Geometry check sheet. Reference: the model listing, model coordinates, mm. A direction names the side the tool comes from. Round coordinates to 2 decimals unless told otherwise and drop trailing zeros. Write each loop counter-clockwise with the first axis right and the second up, starting at its lowest first coordinate (ties: lowest second). Pieces come first, ordered by that corner, then holes.
from build123d import *

# Parameters (mm, degrees)
PAD008_DEPTH    = 3.6
SKETCH034_W     = 6
SKETCH034_H     = 14
SKETCH034_H_2   = 10
POCKET014_DEPTH = 5
FILLET007_R     = 2
SKETCH035_R     = 2.1
POCKET019_DEPTH = 5
SKETCH032_R     = 1.325
POCKET020_DEPTH = 5
SKETCH033_R     = 1.6
HOLE004_DEPTH   = 25
FILLET010_R     = 0.5
POCKET043_DEPTH = 1


with BuildPart() as part:
    # Sketch031 → Pad008 (new body)
    with BuildSketch(Plane.XY):
        Polygon((-12.75, 0), (-12.75, -5), (-12.75, -54), (12.75, -54), (12.75, -5), (12.75, 0), align=None)
    extrude(amount=PAD008_DEPTH)

    # Sketch034 (on Face4 of Pad008) → Pocket014 (cut)
    with BuildSketch(Plane.XY.offset(3.6)):
        with Locations((0, -47)):
            Rectangle(SKETCH034_W, SKETCH034_H)
        with Locations((0, -5)):
            Rectangle(SKETCH034_W, SKETCH034_H_2)
    extrude(amount=-POCKET014_DEPTH, mode=Mode.SUBTRACT)

    # Fillet007
    fillet007_edges = [part.edges().sort_by_distance(p)[0] for p in [
        (-3, -10, 1.8),
        (3, -10, 1.8),
        (3, -40, 1.8),
        (-3, -40, 1.8),
    ]]
    fillet(fillet007_edges, radius=FILLET007_R)

    # Sketch035 (on Face4 of Pad008) → Pocket019 (cut)
    with BuildSketch(Plane.XY.offset(3.6)):
        with Locations((0, -30)):
            Circle(SKETCH035_R)
    extrude(amount=-POCKET019_DEPTH, mode=Mode.SUBTRACT)

    # Sketch032 (on Face4 of Pad008) → Pocket020 (cut)
    with BuildSketch(Plane.XY.offset(3.6)):
        with Locations((-5.7, -24.35)):
            Circle(SKETCH032_R)
        with Locations((5.7, -24.35)):
            Circle(SKETCH032_R)
        with Locations((5.7, -35.65)):
            Circle(SKETCH032_R)
        with Locations((-5.7, -35.65)):
            Circle(SKETCH032_R)
    extrude(amount=-POCKET020_DEPTH, mode=Mode.SUBTRACT)

    # Sketch033 (on Face4 of Pad008) → Hole004 (cut)
    with BuildSketch(Plane.XY.offset(3.6)):
        with Locations((-8, -15)):
            Circle(SKETCH033_R)
        with Locations((8, -15)):
            Circle(SKETCH033_R)
        with Locations((-8, -45)):
            Circle(SKETCH033_R)
        with Locations((8, -45)):
            Circle(SKETCH033_R)
    extrude(amount=-HOLE004_DEPTH, mode=Mode.SUBTRACT)

    # Fillet010
    fillet010_edges = [part.edges().sort_by_distance(p)[0] for p in [
        (-12.75, 0, 1.8),
        (-12.75, -54, 1.8),
        (12.75, 0, 1.8),
        (12.75, -54, 1.8),
    ]]
    fillet(fillet010_edges, radius=FILLET010_R)

    # Sketch098 (on Face31 of Fillet010) → Pocket043 (cut)
    with BuildSketch(Plane.XY.offset(3.6)):
        with BuildLine():
            ThreePointArc((5.7, -21.35), (2.7, -24.35), (5.7, -27.35))
            Line((5.7, -27.35), (12.75, -27.35))
            Line((12.75, -21.35), (12.75, -27.35))
            Line((5.7, -21.35), (12.75, -21.35))
        make_face()
    extrude(amount=-POCKET043_DEPTH, mode=Mode.SUBTRACT)


solid = part.part
1. Access from +Z, -Z, +X, -X, +Y, -Y to the whole of each face (thin tool, end or side, straight path). Record for faces 4 (the face through (0, -40, 2)), 5 (the face through (0, -10, 2)), 6 (the face through (8, 0, 2)).
2. Section check B-B (y = -30). Record the cut outline in (x, z).
3. Section check C-C (x = 0). Record the cut outline in (y, z).
4. Section check D-D (z = 0.95). State how many separate pieces and enclosed holes the cut face has, plus the area to 3 significant figures.
5. Section check A-A (x = -8). Record the cut outline in (y, z).
6. Release check for a two-part mould opening along Y. For faces 1 (the face through (-2.43, -9.4, 1.77)), 2 (the face through (2.7, -24.3, 3.1)), 3 (the face through (2.43, -40.6, 1.77)) record: +Y half, -Y half, draft (parallel to the pull), parting line (faces both ways), or undercut.
7. Depth check by flat-ended pin: pin 1 Ø3.5 at (x, y) = (8, -15) entering from -Z; pin 2 Ø2.5 at (x, y) = (0, -30) entering from -Z; pin 3 Ø1 at (x, z) = (0, 1.5) entering from +Y; pin 4 Ø2 at (x, z) = (0.5, 3) entering from +Y. Enter the tip coordinate at first touch or a pass-through.
8. Scan lines: line 1 along Y through (x, z) = (8, 1.75); line 2 along Y through (x, z) = (5.7, 2.3) (3 decimals); line 3 along Y through (x, z) = (0, 1.7). Record each from-to range of solid material in increasing order.
Results below:
1. face 4: +Z, -Z, -Y
1. face 5: +Z, -Z, +Y
1. face 6: +Z, -Z, +X, -X, +Y
2. outline: (-12.75, 0) - (-2.1, 0) - (-2.1, 3.6) - (-12.75, 3.6) - close; (2.1, 0) - (12.75, 0) - (12.75, 3.6) - (2.1, 3.6) - close
3. outline: (-40, 0) - (-32.1, 0) - (-32.1, 3.6) - (-40, 3.6) - close; (-27.9, 0) - (-10, 0) - (-10, 3.6) - (-27.9, 3.6) - close
4. separate pieces: 1
4. enclosed holes: 9
4. area: 1,170 mm2
5. outline: (-54, 0) - (-46.6, 0) - (-46.6, 3.6) - (-54, 3.6) - close; (-43.4, 0) - (-16.6, 0) - (-16.6, 3.6) - (-43.4, 3.6) - close; (-13.4, 0) - (0, 0) - (0, 3.6) - (-13.4, 3.6) - close
6. face 1: +Y half
6. face 2: undercut
6. face 3: -Y half
7. pin 1: stops at z = 0
7. pin 2: passes through
7. pin 3: stops at y = -10
7. pin 4: stops at y = -9.94
8. line 1: y = -54 to -46.6, -43.4 to -16.6, -13.4 to 0
8. line 2: y = -54 to -36.975, -34.325 to -25.675, -23.025 to 0
8. line 3: y = -40 to -32.1, -27.9 to -10
